Design review of the part shown in the three views and the two pictorial views. Dimensions are in mm from the part's minimum x, y and z. A direction names the side the tool comes from. Round coordinates to 2 decimals unless told otherwise and drop trailing zeros. Loops run counter-clockwise (first coordinate to the right, second up) from the corner with the lowest first, then second, coordinate; pieces in that order, holes last.
1) Take a section at B-B (x = 36.83). State the section outline as (y, z) points (3 decimals), then the cut area to 3 significant figures.
2) Insertion check: pin 1 (12.5 mm diameter, centred on x = 51, z = 15, fed in from -Y); pin 2 (10 mm diameter, centred on y = 4.5, z = 22, fed in from -X). Each pin has a flat end and moves straight along its axis. Give the tip position at first contact, or say it passes through.
3) Take a section at D-D (z = 17.5). State the section outline as (x, y) points, then the cut area to 3 significant figures.
4) Take a section at A-A (z = 12.7). State the section outline as (x, y) points (3 decimals), then the cut area to 3 significant figures.
5) Tool access review of the marked faces 4 and 5: name each direction out of +Z, -Z, +X, -X, +Y, -Y from which nothing blocks a thin tool from reaching the whole face with its end or side.
6) Take a section at C-C (y = 16.5). State the section outline as (x, z) points.
7) Wall thickness on L1, parallel to X at y = 16, z = 10.75; L2, parallel to Z at x = 36.83, y = 24.45 (3 decimals); L3, parallel to Y at x = 55, z = 12.75: over which ranges is each line inside the solid? List them lowest first.
8) Mouldability with a two-part tool opening along X and no side actions: class the marked faces 1, 2 and 3 as pulls with the +X half, pulls with the -X half, needs draft (parallel to the pull), parting line crosses it, or undercut.
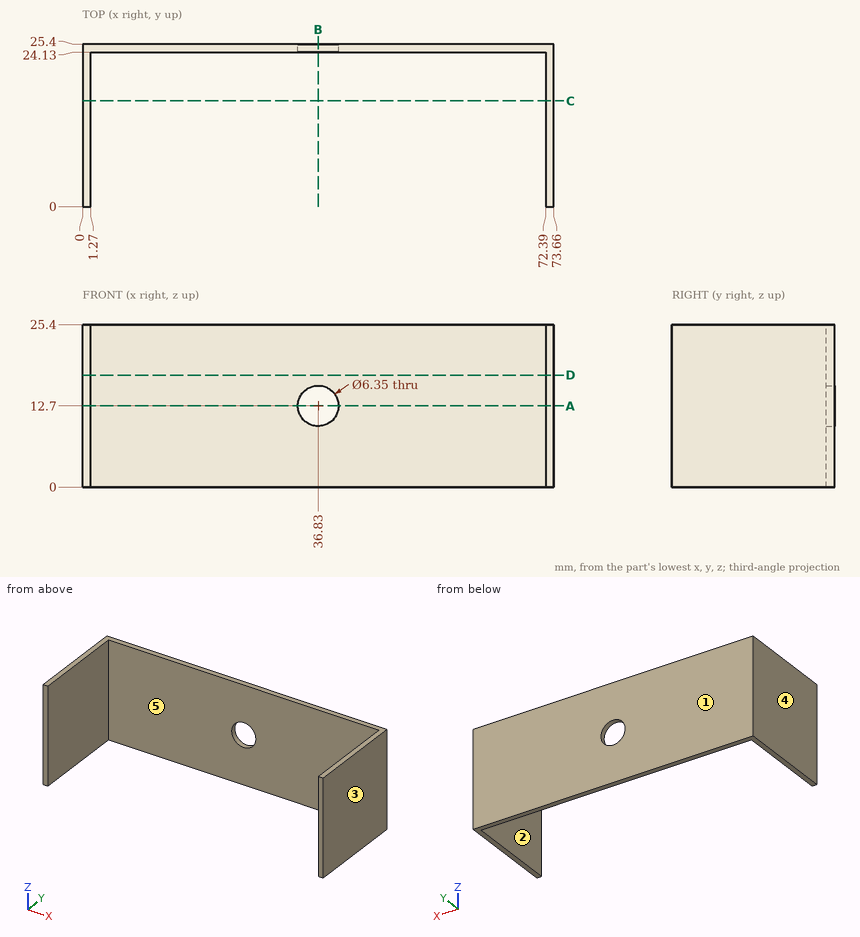
Response:
1. outline: (24.13, 0) - (25.4, 0) - (25.4, 9.525) - (24.13, 9.525) - close; (24.13, 15.875) - (25.4, 15.875) - (25.4, 25.4) - (24.13, 25.4) - close
1. area: 24.2 mm2
2. pin 1: stops at y = 24.13
2. pin 2: stops at x = 0
3. outline: (0, 0) - (1.27, 0) - (1.27, 24.13) - (72.39, 24.13) - (72.39, 0) - (73.66, 0) - (73.66, 25.4) - (0, 25.4) - close
3. area: 155 mm2
4. outline: (0, 0) - (1.27, 0) - (1.27, 24.13) - (33.655, 24.13) - (33.655, 25.4) - (0, 25.4) - close; (40.005, 24.13) - (72.39, 24.13) - (72.39, 0) - (73.66, 0) - (73.66, 25.4) - (40.005, 25.4) - close
4. area: 147 mm2
5. face 4: +Z, -Z, -X, +Y, -Y
5. face 5: +Z, -Z, -Y
6. outline: (0, 0) - (1.27, 0) - (1.27, 25.4) - (0, 25.4) - close; (72.39, 0) - (73.66, 0) - (73.66, 25.4) - (72.39, 25.4) - close
7. L1: x = 0 to 1.27, 72.39 to 73.66
7. L2: z = 0 to 9.525, 15.875 to 25.4
7. L3: y = 24.13 to 25.4
8. face 1: needs draft
8. face 2: undercut
8. face 3: pulls with the +X half
